from build123d import *

# Parameters (mm, degrees)
ESQUISSE1_W             = 154
ESQUISSE1_H             = 101
BOSS_EXTRU_1_DEPTH      = 5
ESQUISSE2_R             = 16
ESQUISSE2_R_2           = 1.5
ENL_V_MAT_EXTRU_2_DEPTH = 5
ESQUISSE3_R             = 1.5
ENL_V_MAT_EXTRU_3_DEPTH = 5
ESQUISSE8_W             = 164
ESQUISSE8_H             = 113
ESQUISSE8_W_2           = 154
ESQUISSE8_H_2           = 103
BOSS_EXTRU_3_DEPTH      = 53
BOSS_EXTRU_3_DEPTH_BACK = 5
ESQUISSE9_W             = 154
ESQUISSE9_H             = 2
BOSS_EXTRU_4_DEPTH      = 5
ESQUISSE11_W            = 70
ESQUISSE11_H            = 5
ENL_V_MAT_EXTRU_7_DEPTH = 38
ESQUISSE12_W            = 50
ESQUISSE12_H            = 5
ESQUISSE12_W_2          = 5
ESQUISSE12_H_2          = 50
ENL_V_MAT_EXTRU_8_DEPTH = 5
ESQUISSE13_W            = 25
ESQUISSE13_H            = 5
ENL_V_MAT_EXTRU_9_DEPTH = 5


with BuildPart() as part:
    # Esquisse1 → Boss.-Extru.1 (new body)
    with BuildSketch(Plane(origin=(0, 0, 0), x_dir=(1, 0, 0), z_dir=(0, 1, 0))):
        Rectangle(ESQUISSE1_W, ESQUISSE1_H)
    extrude(amount=BOSS_EXTRU_1_DEPTH)

    # Esquisse2 → Enlèv. mat.-Extru.2 (cut)
    with BuildSketch(Plane(origin=(0, 5, 0), x_dir=(1, 0, 0), z_dir=(0, 1, 0))):
        Circle(ESQUISSE2_R)
        with Locations((0, 21)):
            Circle(ESQUISSE2_R_2)
        with Locations((-21, 0)):
            Circle(ESQUISSE2_R_2)
        with Locations((21, 0)):
            Circle(ESQUISSE2_R_2)
        with Locations((0, -21)):
            Circle(ESQUISSE2_R_2)
    extrude(amount=-ENL_V_MAT_EXTRU_2_DEPTH, mode=Mode.SUBTRACT)

    # Esquisse3 → Enlèv. mat.-Extru.3 (cut)
    with BuildSketch(Plane(origin=(0, 5, 0), x_dir=(1, 0, 0), z_dir=(0, 1, 0))):
        with Locations((70, -45.5)):
            Circle(ESQUISSE3_R)
        with Locations((-70, -45.5)):
            Circle(ESQUISSE3_R)
        with Locations((-70, 42.5)):
            Circle(ESQUISSE3_R)
        with Locations((70, 42.5)):
            Circle(ESQUISSE3_R)
    extrude(amount=-ENL_V_MAT_EXTRU_3_DEPTH, mode=Mode.SUBTRACT)



with BuildPart() as body_2:
    # Esquisse8 → Boss.-Extru.3 (new body, two sides)
    with BuildSketch(Plane(origin=(0, 5, 0), x_dir=(1, 0, 0), z_dir=(0, 1, 0))) as boss_extru_3_sk:
        with Locations((0, -1)):
            Rectangle(ESQUISSE8_W, ESQUISSE8_H)
        with Locations((0, -1)):
            Rectangle(ESQUISSE8_W_2, ESQUISSE8_H_2, mode=Mode.SUBTRACT)
    extrude(amount=BOSS_EXTRU_3_DEPTH)
    extrude(boss_extru_3_sk.sketch, amount=-BOSS_EXTRU_3_DEPTH_BACK)


with BuildPart() as part_1:
    add(part.part)

    add(body_2.part)  # Boss.-Extru.4 merges body 2
    # Esquisse9 → Boss.-Extru.4 (add)
    with BuildSketch(Plane(origin=(0, 0, 0), x_dir=(-1, 0, 0), z_dir=(0, -1, 0))):
        with Locations((0, -51.5)):
            Rectangle(ESQUISSE9_W, ESQUISSE9_H)
    extrude(amount=-BOSS_EXTRU_4_DEPTH)

    # Esquisse11 → Enlèv. mat.-Extru.7 (cut)
    with BuildSketch(Plane(origin=(0, 58, 0), x_dir=(1, 0, 0), z_dir=(0, 1, 0))):
        with Locations((-24.3, -55)):
            Rectangle(ESQUISSE11_W, ESQUISSE11_H)
    extrude(amount=-ENL_V_MAT_EXTRU_7_DEPTH, mode=Mode.SUBTRACT)

    # Esquisse12 → Enlèv. mat.-Extru.8 (cut)
    with BuildSketch(Plane(origin=(0, 58, 0), x_dir=(1, 0, 0), z_dir=(0, 1, 0))):
        with Locations((0, 53)):
            Rectangle(ESQUISSE12_W, ESQUISSE12_H)
        with Locations((79.5, -1)):
            Rectangle(ESQUISSE12_W_2, ESQUISSE12_H_2)
        with Locations((-79.5, -1)):
            Rectangle(ESQUISSE12_W_2, ESQUISSE12_H_2)
    extrude(amount=-ENL_V_MAT_EXTRU_8_DEPTH, mode=Mode.SUBTRACT)

    # Esquisse13 → Enlèv. mat.-Extru.9 (cut)
    with BuildSketch(Plane(origin=(0, 58, 0), x_dir=(1, 0, 0), z_dir=(0, 1, 0))):
        with Locations((46.35, -55)):
            Rectangle(ESQUISSE13_W, ESQUISSE13_H)
    extrude(amount=-ENL_V_MAT_EXTRU_9_DEPTH, mode=Mode.SUBTRACT)


solid = part_1.part
Check sheet for the modelled part. Datum: model origin and axes. Units: mm. A direction names the side the tool comes from. Round coordinates to 2 decimals unless told otherwise and drop trailing zeros. Order: outer loops, then holes, each group sorted by start corner. A loop starts at its lowest first (then second) coordinate and runs counter-clockwise, first axis right, second up.
Q1. Cross-section at B-B, the plane y = 12. Enter the section's corners in (x, z), plus the area to 3 significant figures.
Filled sheet:
outline: (-82, -55.5) - (82, -55.5) - (82, 57.5) - (-82, 57.5) - close; hole (-77, -50.5) - (77, -50.5) - (77, 52.5) - (-77, 52.5) - close
area: 2,670 mm2
Q2. Cross-section at C-C, the plane x = 48. Enter the section's corners in (y, z).
Filled sheet:
outline: (0, -55.5) - (58, -55.5) - (58, -50.5) - (5, -50.5) - (5, 52.5) - (53, 52.5) - (53, 57.5) - (0, 57.5) - close
Q3. Scan lines: L1, parallel to X at y = 2.3, z = 0; L2, parallel to Z at x = -61.5, y = 44; L3, parallel to X at y = 20, z = -3. Record each from-to range of solid material in increasing order.
Filled sheet:
L1: x = -82 to -22.5, -19.5 to -16, 16 to 19.5, 22.5 to 82
L2: z = -55.5 to -50.5, 52.5 to 57.5
L3: x = -82 to -77, 77 to 82
Q4. Set-up check for faces 1 (the face through (-1, 32, -50.5)), 2 (the face through (-25, 56, -53)), 3 (the face through (-80, 56, 26)): record each of +Z, -Z, +X, -X, +Y, -Y from which the full face is reachable in a straight line by a thin tool's end or side.
Filled sheet:
face 1: +Y
face 2: +Z, -Z, +Y
face 3: +X, -X, +Y
Q5. Cross-section at D-D, the plane z = -35. Enter the section's corners in (x, y).
Filled sheet:
outline: (-82, 0) - (82, 0) - (82, 58) - (77, 58) - (77, 5) - (-77, 5) - (-77, 58) - (-82, 58) - close
Q6. Draft check along X on faces 4 (the face through (-82, 29, 2)), 5 (the face through (-1, 29, -55.5)), 6 (the face through (82, 29, 2)), 7 (the face through (46, 53, 55)). Enter one of: pulls with the +X half, pulls with the -X half, needs draft (parallel to the pull), parting line crosses it, or undercut.
Filled sheet:
face 4: pulls with the -X half
face 5: needs draft
face 6: pulls with the +X half
face 7: undercut
Q7. Depth check by flat-ended pin: P1, Ø6, axis at x = 47.5, z = -15, coming from the +Y side; P2, Ø5.5, axis at x = -79, z = -3.5, coming from the +Y side; P3, Ø2.5, axis at x = 21, z = 0, coming from the +Y side; P4, Ø12, axis at x = -41.5, y = 36, coming from the +Z side. Enter the tip coordinate at first touch or a pass-through.
Filled sheet:
P1: stops at y = 5
P2: stops at y = 53
P3: passes through
P4: stops at z = -50.5
Q8. Cross-section at A-A, the plane z = 10. Enter the section's corners in (x, y).
Filled sheet:
outline: (-82, 0) - (-12.49, 0) - (-12.49, 5) - (-77, 5) - (-77, 53) - (-82, 53) - close; (12.49, 0) - (82, 0) - (82, 53) - (77, 53) - (77, 5) - (12.49, 5) - close
